from build123d import *

# Parameters (mm, degrees)
SKETCH1_R               = 31
SKETCH1_R_2             = 29
BOSS_EXTRUDE1_DEPTH     = 140
CUT_EXTRUDE1_DEPTH      = 147.703783182
CUT_EXTRUDE1_DEPTH_BACK = 147.703783182
SKETCH2_R               = 1.5
CUT_EXTRUDE2_DEPTH      = 147.703783323
CUT_EXTRUDE2_DEPTH_BACK = 147.703783323
SKETCH3_R               = 1.5


with BuildPart() as part:
    # Sketch1 → Boss-Extrude1 (new body)
    with BuildSketch(Plane(origin=(0, 0, 0), x_dir=(1, 0, 0), z_dir=(0, 1, 0))):
        with Locations(Location((0, 0, 0), (0, 0, 270))):
            Circle(SKETCH1_R)
        with Locations(Location((0, 0, 0), (0, 0, 270))):
            Circle(SKETCH1_R_2, mode=Mode.SUBTRACT)
    extrude(amount=BOSS_EXTRUDE1_DEPTH)

    # Sketch2 → Cut-Extrude1 (cut, two sides: drawn at the far end of the back side and taken through both)
    with BuildSketch(Plane(origin=(0, 0, 0), x_dir=(0, 0, -1), z_dir=(1, 0, 0)).offset(-CUT_EXTRUDE1_DEPTH_BACK)):
        with Locations((0, 33.088409151)):
            Circle(SKETCH2_R)
        with Locations((0, 106.088409151)):
            Circle(SKETCH2_R)
    extrude(amount=CUT_EXTRUDE1_DEPTH + CUT_EXTRUDE1_DEPTH_BACK, mode=Mode.SUBTRACT)

    # Sketch3 → Cut-Extrude2 (cut, two sides: drawn at the far end of the back side and taken through both)
    with BuildSketch(Plane.XY.offset(-CUT_EXTRUDE2_DEPTH_BACK)):
        with Locations((0, 106.088379232)):
            Circle(SKETCH3_R)
        with Locations((0, 33.5)):
            Circle(SKETCH3_R)
    extrude(amount=CUT_EXTRUDE2_DEPTH + CUT_EXTRUDE2_DEPTH_BACK, mode=Mode.SUBTRACT)


solid = part.part
Source: CAD feature listing. Evaluate the final solid. Frame: model axes, mm. Round coordinates to 2 decimals unless told otherwise and drop trailing zeros. Write each loop counter-clockwise with the first axis right and the second up, starting at its lowest first coordinate (ties: lowest second). Pieces come first, ordered by that corner, then holes. Notation, with made-up numbers: M -4.75,44.5 L 6.25,44.5 A22 cw 6.25,50.5 Z; hole C -35,5.5 d3. An arc over 180 degrees is marked long. One line per item, written item: value. Start each with the question number.
Item 1: Section query C-C (x = -20). Return the cut outline in (y, z), plus the area to 3 significant figures.
Item 2: Section query A-A (x = 0). Return the cut outline in (y, z), plus the area to 3 significant figures.
Item 3: Mould query, pull axis Y, two halves, no side actions, for faces 1 (the cylindrical face through (29.966, 34.576, 0.195)), 2 (the flat face through (-21, 0, 21)), 3 (the flat face through (-21, 140, 21)). Classes: pulls with the +Y half, pulls with the -Y half, needs draft (parallel to the pull), parting line crosses it, or undercut.
Item 4: Ray query, L1, parallel to Y at x = 0, z = 30; L2, parallel to Z at x = -8, y = 10.5; L3, parallel to Z at x = -22, y = 31.5. Return the intervals inside material, ascending. Write a range as from..to.
Item 5: Pin query (flat end, axial travel): pin 1 (4 mm diameter, centred on y = 20, z = 11, fed in from -X); pin 2 (2 mm diameter, centred on y = 34, z = -9.5, fed in from +X); pin 3 (2.5 mm diameter, centred on x = 0, y = 106.09, fed in from -Z); pin 4 (12 mm diameter, centred on x = 18.5, y = 68.5, fed in from +Z). Return the tip coordinate at first contact, or that it passes through.
Item 6: Section query D-D (z = 25). Return the cut outline in (x, y).
Item 7: Section query B-B (z = 0). Return the cut outline in (x, y).
Result set:
1. outline: M 0,-23.69 L 140,-23.69 L 140,-21 L 0,-21 Z; M 0,21 L 140,21 L 140,23.69 L 0,23.69 Z
1. area: 752 mm²
2. outline: M 0,-31 L 32,-31 L 32,-29 L 0,-29 Z; M 0,29 L 32,29 L 32,31 L 0,31 Z; M 35,-31 L 104.59,-31 L 104.59,-29 L 35,-29 Z; M 35,29 L 104.59,29 L 104.59,31 L 35,31 Z; M 107.59,-31 L 140,-31 L 140,-29 L 107.59,-29 Z; M 107.59,29 L 140,29 L 140,31 L 107.59,31 Z
2. area: 536 mm²
3. face 1: undercut
3. face 2: pulls with the -Y half
3. face 3: pulls with the +Y half
4. L1: y = 0..32, 35..104.59, 107.59..140
4. L2: z = -29.95..-27.87, 27.87..29.95
4. L3: z = -21.84..-18.89, 18.89..21.84
5. pin 1: stops at x = -29.66
5. pin 2: stops at x = 29.81
5. pin 3: passes through
5. pin 4: stops at z = 28.37
6. outline: M -18.33,0 L -14.7,0 L -14.7,140 L -18.33,140 Z; M 14.7,0 L 18.33,0 L 18.33,140 L 14.7,140 Z
7. outline: M -31,0 L -29,0 L -29,31.59 L -31,31.59 Z; M -31,34.59 L -29,34.59 L -29,104.59 L -31,104.59 Z; M -31,107.59 L -29,107.59 L -29,140 L -31,140 Z; M 29,0 L 31,0 L 31,31.59 L 29,31.59 Z; M 29,34.59 L 31,34.59 L 31,104.59 L 29,104.59 Z; M 29,107.59 L 31,107.59 L 31,140 L 29,140 Z
